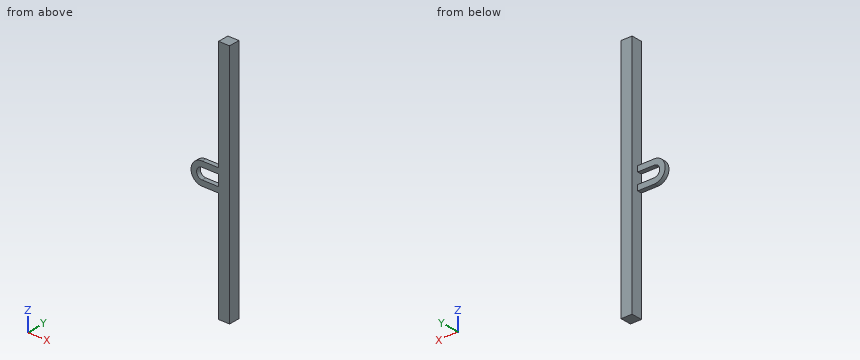
from build123d import *

# Parameters (mm, degrees)
SKETCH1_W           = 12.7
SKETCH1_H           = 279.4
BOSS_EXTRUDE1_DEPTH = 12.7
BOSS_EXTRUDE2_DEPTH = 5.08


with BuildPart() as part:
    # Sketch1 → Boss-Extrude1 (new body)
    with BuildSketch(Plane(origin=(0, 0, 0), x_dir=(1, 0, 0), z_dir=(0, 1, 0))):
        Rectangle(SKETCH1_W, SKETCH1_H)
    extrude(amount=BOSS_EXTRUDE1_DEPTH)

    # Sketch1_4 → Boss-Extrude2 (add)
    with BuildSketch(Plane(origin=(0, 0, 0), x_dir=(1, 0, 0), z_dir=(0, 1, 0))):
        with BuildLine():
            Line((-14.401477372, 6.35), (-6.35, 6.35))
            Line((-6.35, 6.35), (-6.35, 12.7))
            Line((-6.35, 12.7), (-25.4, 12.7))
            ThreePointArc((-25.4, 12.7), (-19.05, 10.998522628), (-14.401477372, 6.35))
        make_face()
        with BuildLine():
            ThreePointArc((-25.4, 12.7), (-38.1, 0), (-25.4, -12.7))
            ThreePointArc((-25.4, -12.7), (-19.05, -10.998522628), (-14.401477372, -6.35))
            Line((-14.401477372, -6.35), (-25.4, -6.35))
            ThreePointArc((-25.4, -6.35), (-31.75, 0), (-25.4, 6.35))
            Line((-25.4, 6.35), (-14.401477372, 6.35))
            ThreePointArc((-14.401477372, 6.35), (-19.05, 10.998522628), (-25.4, 12.7))
        make_face()
        with BuildLine():
            Line((-25.4, -12.7), (-6.35, -12.7))
            Line((-6.35, -12.7), (-6.35, -6.35))
            Line((-6.35, -6.35), (-14.401477372, -6.35))
            ThreePointArc((-14.401477372, -6.35), (-19.05, -10.998522628), (-25.4, -12.7))
        make_face()
    extrude(amount=BOSS_EXTRUDE2_DEPTH)


solid = part.part
Verification items for the finished model (mm, model axes). Coordinates: 2 decimals unless noted, no trailing zeros. Order: outer loops, then holes, each group sorted by start corner. A loop starts at its lowest first (then second) coordinate and runs counter-clockwise, first axis right, second up. Notation, with made-up numbers: M 78,5.5 L 134,5.5 A28 cw 134,39.5 Z; hole C 29,-9 d11. An arc over 180 degrees is marked long. Return JSON: item names as keys, results as strings.
1) Cross-section at D-D, the plane z = 53. Record the boundary of the cut face in (x, y), and give its area (3 significant figures).
Answer list:
{"outline": "M -6.35,0 L 6.35,0 L 6.35,12.7 L -6.35,12.7 Z", "area": "161 mm2"}
2) Cross-section at A-A, the plane z = 0. Record the boundary of the cut face in (x, y).
Answer list:
{"outline": "M -38.1,0 L -31.75,0 L -31.75,5.08 L -38.1,5.08 Z; M -6.35,0 L 6.35,0 L 6.35,12.7 L -6.35,12.7 Z"}
3) Cross-section at C-C, the plane y = 10.5. Record the boundary of the cut face in (x, z), and give its area (3 significant figures).
Answer list:
{"outline": "M -6.35,-139.7 L 6.35,-139.7 L 6.35,139.7 L -6.35,139.7 Z", "area": "3,550 mm2"}
4) Thickness scan on L1, parallel to X at y = 4.5, z = -0.5; L2, parallel to Z at x = -15, y = 3; L3, parallel to Z at x = -30, y = 4.25. Record the ranges inside material, lowest first. Write a range as [from, to].
Answer list:
{"L1": "[-38.09, -31.73], [-6.35, 6.35]", "L2": "[-12.7, -6.35], [6.35, 12.7]", "L3": "[-11.84, -4.38], [4.38, 11.84]"}
5) Gauge pin test, flat ends, axial feed: pin 1 (1.5 mm diameter, centred on x = -4.5, z = 60, fed in from -Y); pin 2 (2.5 mm diameter, centred on x = -17, y = 1.5, fed in from -Z); pin 3 (4 mm diameter, centred on x = -14.5, y = 2, fed in from +Z); pin 4 (3 mm diameter, centred on y = 6, z = 6.5, fed in from -X). Record the tip position at first contact, or that the pin passes through.
Answer list:
{"pin 1": "y = 0", "pin 2": "z = -12.7", "pin 3": "z = 12.7", "pin 4": "x = -36.93"}
6) Cross-section at B-B, the plane x = -16. Record the boundary of the cut face in (y, z).
Answer list:
{"outline": "M 0,-12.7 L 5.08,-12.7 L 5.08,-6.35 L 0,-6.35 Z; M 0,6.35 L 5.08,6.35 L 5.08,12.7 L 0,12.7 Z"}
